```python
from build123d import *

# Parameters (mm, degrees)
F0_W     = 42
F0_H     = 74
F0_R     = 1.75
F1_DEPTH = 6
F3_R     = 5
F2_R     = 3
F4_DEPTH = 3
F5_R     = 2.75
F6_DEPTH = 6
F7_R     = 4.75
F8_DEPTH = 2


with BuildPart() as f1:
    # F0 (on Front) → F1 (new body)
    with BuildSketch(Plane.XZ):
        Rectangle(F0_W, F0_H)
        with Locations((-15.75, 0.75)):
            Circle(F0_R, mode=Mode.SUBTRACT)
        with Locations((-15.75, 31.75)):
            Circle(F0_R, mode=Mode.SUBTRACT)
        with Locations((15.75, 0.75)):
            Circle(F0_R, mode=Mode.SUBTRACT)
        with Locations((15.75, 31.75)):
            Circle(F0_R, mode=Mode.SUBTRACT)
    extrude(amount=F1_DEPTH)

    # F3
    f3_edges = [f1.edges().sort_by_distance(p)[0] for p in [
        (-21, -3, -37),
        (-21, -3, 37),
        (21, -3, 37),
        (21, -3, -37),
    ]]
    fillet(f3_edges, radius=F3_R)

    # F2 (on face) → F4 (cut)
    with BuildSketch(Plane.XZ.offset(6)):
        with Locations((-15.75, 0.75)):
            Circle(F2_R)
        with Locations((15.75, 0.75)):
            Circle(F2_R)
        with Locations((-15.75, 31.75)):
            Circle(F2_R)
        with Locations((15.75, 31.75)):
            Circle(F2_R)
    extrude(amount=-F4_DEPTH, mode=Mode.SUBTRACT)

    # F5 (on face) → F6 (cut, through all)
    with BuildSketch(Plane.XZ.offset(6)):
        with Locations((0, -22)):
            Circle(F5_R)
        with Locations((-10, -12)):
            Circle(F5_R)
        with Locations((10, -12)):
            Circle(F5_R)
    extrude(amount=-F6_DEPTH, mode=Mode.SUBTRACT)

    # F7 (on face) → F8 (cut)
    with BuildSketch(Plane(origin=(0, 0, 0), x_dir=(-1, 0, 0), z_dir=(0, 1, 0))):
        with Locations((-10, -12)):
            Circle(F7_R)
        with Locations((10, -12)):
            Circle(F7_R)
        with Locations((0, -22)):
            Circle(F7_R)
    extrude(amount=-F8_DEPTH, mode=Mode.SUBTRACT)


solid = f1.part
```
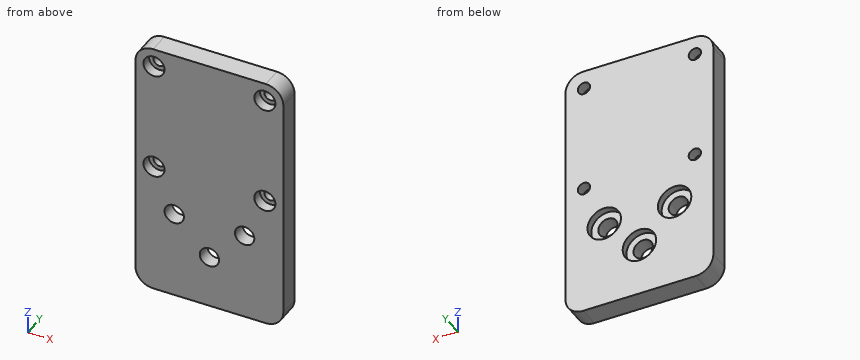
For this review, take the finished solid that the model builds, in its own axes (mm). Round coordinates to 2 decimals unless told otherwise and drop trailing zeros. Write each loop counter-clockwise with the first axis right and the second up, starting at its lowest first coordinate (ties: lowest second). Pieces come first, ordered by that corner, then holes.
1) For line 1 along Z through (x, y) = (-15.75, -1.55); line 2 along X through (y, z) = (-1.7, 0.75); line 3 along Z through (x, y) = (10, -3.6), list the stretches that pass through material, from the lowest coordinate up.
Answer below:
line 1: z = -37 to -1, 2.5 to 30, 33.5 to 37
line 2: x = -21 to -17.5, -14 to 14, 17.5 to 21
line 3: z = -37 to -14.75, -9.25 to 37
2) Insertion check: pin 1 Ø3 at (x, z) = (0, -23.5) entering from +Y; pin 2 Ø5 at (x, z) = (-15.75, 0.75) entering from -Y. Each pin has a flat end and moves straight along its axis. Give the tip position at first contact, or say it passes through.
Answer below:
pin 1: stops at y = -2
pin 2: stops at y = -3
3) Take a section at D-D on z = 0.75. Give the boundary of the cut face in (x, y), then the cut area to 3 significant figures.
Answer below:
outline: (-21, -6) - (-18.75, -6) - (-18.75, -3) - (-17.5, -3) - (-17.5, 0) - (-21, 0) - close; (-14, -3) - (-12.75, -3) - (-12.75, -6) - (12.75, -6) - (12.75, -3) - (14, -3) - (14, 0) - (-14, 0) - close; (17.5, -3) - (18.75, -3) - (18.75, -6) - (21, -6) - (21, 0) - (17.5, 0) - close
area: 195 mm2
4) Take a section at C-C on y = -3.7. Give the boundary of the cut face in (x, z).
Answer below:
outline: (-21, -32) arc R5 ccw to (-16, -37) - (16, -37) arc R5 ccw to (21, -32) - (21, 32) arc R5 ccw to (16, 37) - (-16, 37) arc R5 ccw to (-21, 32) - close; hole circle Ø6 at (-15.75, 0.75); hole circle Ø6 at (-15.75, 31.75); hole circle Ø5.5 at (-10, -12); hole circle Ø5.5 at (0, -22); hole circle Ø5.5 at (10, -12); hole circle Ø6 at (15.75, 0.75); hole circle Ø6 at (15.75, 31.75)
5) Take a section at A-A on z = -12. Give the boundary of the cut face in (x, y), then the cut area to 3 significant figures.
Answer below:
outline: (-21, -6) - (-12.75, -6) - (-12.75, -2) - (-14.75, -2) - (-14.75, 0) - (-21, 0) - close; (-7.25, -6) - (7.25, -6) - (7.25, -2) - (5.25, -2) - (5.25, 0) - (-5.25, 0) - (-5.25, -2) - (-7.25, -2) - close; (12.75, -6) - (21, -6) - (21, 0) - (14.75, 0) - (14.75, -2) - (12.75, -2) - close
area: 170 mm2
6) Take a section at B-B on x = 0. Give the boundary of the cut face in (y, z).
Answer below:
outline: (-6, -37) - (0, -37) - (0, -26.75) - (-2, -26.75) - (-2, -24.75) - (-6, -24.75) - close; (-6, -19.25) - (-2, -19.25) - (-2, -17.25) - (0, -17.25) - (0, 37) - (-6, 37) - close
